```python
from build123d import *

# Parameters (mm, degrees)
SALIENTE_EXTRUIR1_DEPTH      = 14
SALIENTE_EXTRUIR3_DEPTH      = 9
SALIENTE_EXTRUIR3_DEPTH_BACK = 5
CROQUIS5_R                   = 2.85
CORTAR_EXTRUIR3_DEPTH        = 6.5
CORTAR_EXTRUIR4_DEPTH        = 21
CROQUIS7_R                   = 1
CORTAR_EXTRUIR5_DEPTH        = 5
CROQUIS8_R                   = 0.94
CORTAR_EXTRUIR6_DEPTH        = 45.465042449
REDONDEO2_R                  = 5
REDONDEO3_R                  = 2


with BuildPart() as part:
    # Croquis1 → Saliente-Extruir1 (new body)
    with BuildSketch(Plane(origin=(0, 0, 0), x_dir=(1, 0, 0), z_dir=(0, 1, 0))):
        Polygon((0, 0), (5, 0), (5, 19.2), (10, 22.7), (10, 41.7), (5, 41.7), (5, 26.2), (0, 22.7), align=None)
    extrude(amount=SALIENTE_EXTRUIR1_DEPTH)

    # Croquis2 → Saliente-Extruir3 (add, two sides: drawn at the far end of the back side and taken through both)
    with BuildSketch(Plane.XY.offset(-SALIENTE_EXTRUIR3_DEPTH_BACK)):
        Polygon((0, 0), (0, 2), (5, 2), (5, 14), (10, 14), (10, 0), align=None)
    extrude(amount=SALIENTE_EXTRUIR3_DEPTH + SALIENTE_EXTRUIR3_DEPTH_BACK)

    # Croquis5 → Cortar-Extruir3 (cut)
    with BuildSketch(Plane.ZY):
        with Locations((6.7, 7.28)):
            Circle(CROQUIS5_R)
    extrude(amount=-CORTAR_EXTRUIR3_DEPTH, mode=Mode.SUBTRACT)

    # Croquis6 → Cortar-Extruir4 (cut)
    with BuildSketch(Plane.XY.offset(9)):
        with BuildLine():
            Line((5, 0), (10, 0))
            Line((10, 0), (10, 5.596996732))
            ThreePointArc((10, 5.596996732), (8.187050213, 2.184731514), (5, 0))
        make_face()
    extrude(amount=-CORTAR_EXTRUIR4_DEPTH, mode=Mode.SUBTRACT)

    # Croquis7 → Cortar-Extruir5 (cut)
    with BuildSketch(Plane.XZ):
        with Locations(Location((7.5, -37, 0), (0, 0, 270))):
            Circle(CROQUIS7_R)
        with Locations(Location((2.5, -5.1, 0), (0, 0, 270))):
            Circle(CROQUIS7_R)
    extrude(amount=-CORTAR_EXTRUIR5_DEPTH, mode=Mode.SUBTRACT)

    # Croquis8 → Cortar-Extruir6 (cut, through all)
    with BuildSketch(Plane.ZY.offset(-6.5)):
        with Locations((6.7, 7.28)):
            Circle(CROQUIS8_R)
    extrude(amount=-CORTAR_EXTRUIR6_DEPTH, mode=Mode.SUBTRACT)

    # Redondeo2
    redondeo2_edges = [part.edges().sort_by_distance(p)[0] for p in [
        (0, 8, 0),
    ]]
    fillet(redondeo2_edges, radius=REDONDEO2_R - 0.0001)  # a hair under: the kernel refuses the full size

    # Redondeo3
    redondeo3_edges = [part.edges().sort_by_distance(p)[0] for p in [
        (5, 2, 4.5),
    ]]
    fillet(redondeo3_edges, radius=REDONDEO3_R)


solid = part.part
```
Can you work these out from the model? Positions are in its coordinate system, mm. A direction names the side the tool comes from. Coordinates: 2 decimals unless noted, no trailing zeros. Order: outer loops, then holes, each group sorted by start corner. A loop starts at its lowest first (then second) coordinate and runs counter-clockwise, first axis right, second up. Notation, with made-up numbers: (2.25, 19.5) - (6.25, 19.5) arc R16 ccw to (6.25, 49.5) - close; hole circle Ø6 at (47.5, -23). An arc over 180 degrees is marked (long way). Answer in a Markdown table with one row per item.
1. Suppose I cut it at D-D (z = -37). Please give me the cut outline in (x, y).
Reply:
| item | result |
|---|---|
| outline | (5, 0) - (6.5, 0) - (6.5, 5) - (8.5, 5) - (8.5, 0) - (10, 0) - (10, 14) - (5, 14) - close |
2. Suppose I cut it at C-C (x = 6). Please give me the cut outline in (y, z).
Reply:
| item | result |
|---|---|
| outline | (0, -41.7) - (14, -41.7) - (14, -19.9) - (0, -19.9) - close; (0.46, -5) - (14, -5) - (14, 9) - (8.96, 9) arc R2.85 cw (long way) to (5.6, 9) - (0.46, 9) - close |
3. For pin 1 (3 mm diameter, centred on y = 7.28, z = 6.7, fed in from -X); pin 2 (1 mm diameter, centred on y = 12.5, z = -21, fed in from +X); pin 3 (7 mm diameter, centred on y = 8, z = -36, fed in from -X), each with a flat end and sliding along its axis, tell me the tip position at first contact or that it passes through.
Reply:
| item | result |
|---|---|
| pin 1 | stops at x = 6.5 |
| pin 2 | stops at x = 8.29 |
| pin 3 | stops at x = 5 |
4. If I drill on line 1 along Z through (x, y) = (5.25, 4.75) (3 decimals); line 2 along X through (y, z) = (1.5, -27); line 3 along Z through (x, y) = (5.25, 2) (3 decimals), over which ranges is the centre line in solid material (lowest first)?
Reply:
| item | result |
|---|---|
| line 1 | z = -41.7 to -19.375, -5 to 5.388, 8.012 to 9 |
| line 2 | x = 5 to 10 |
| line 3 | z = -41.7 to -19.375, -5 to 9 |
5. Suppose I cut it at A-A (z = 6.7). Please give me the cut outline in (x, y).
Reply:
| item | result |
|---|---|
| outline | (0, 0) - (5, 0) arc R8.1 ccw to (10, 5.6) - (10, 6.34) - (6.5, 6.34) - (6.5, 4.43) - (5, 4.43) - (5, 4) arc R2 cw to (3, 2) - (0, 2) - close; (5, 10.13) - (6.5, 10.13) - (6.5, 8.22) - (10, 8.22) - (10, 14) - (5, 14) - close |
6. If we mould it in two halves opening along Z, with no side actions, what happens to faces 1 (the flat face through (8, 7, -41.7)), 2 (the flat face through (8, 7, -5)), 3 (the flat face through (7, 7, 9)), 4 (the flat face through (1, 2, 3))? For each: pulls with the +Z half, pulls with the -Z half, needs draft (parallel to the pull), parting line crosses it, or undercut.
Reply:
| item | result |
|---|---|
| face 1 | pulls with the -Z half |
| face 2 | undercut |
| face 3 | pulls with the +Z half |
| face 4 | needs draft |
7. For faces 5 (the cylindrical face through (3.49, 2.46, -4.97)), 6 (the cylindrical face through (5.74, 7.38, 3.85)), 7 (the flat face through (7.465, 6.902, -20.926)), 8 (the cylindrical face through (8.2, 2.2, 2.1)), 9 (the cylindrical face through (4.43, 2.6, 4.36)), which set-ups out of +Z, -Z, +X, -X, +Y, -Y let a thin tool reach every point of the face, with its end or its side?
Reply:
| item | result |
|---|---|
| face 5 | -Y |
| face 6 | -X |
| face 7 | +X, +Y, -Y |
| face 8 | +Z, +X, -Y |
| face 9 | +Z, -X, +Y |
